Source: CAD feature listing. Evaluate the final solid. Frame: model axes, mm. A direction names the side the tool comes from. Give positions to 0.01 mm unless a question says otherwise; leave off trailing zeros. Write each loop counter-clockwise with the first axis right and the second up, starting at its lowest first coordinate (ties: lowest second). Pieces come first, ordered by that corner, then holes. Notation, with made-up numbers: (-4.75, -29.75) -> (14.25, -29.75) arc R25 cw to (14.25, 9.25) -> close; hole circle Ø3 at (35, -28.5). An arc over 180 degrees is marked (long way). Use one line per item in the form item = value. Start each with the question number.
(1) Material intervals for line 1 along Y through (x, z) = (-18.5, 1.25); line 2 along Y through (x, z) = (-26, 4.25); line 3 along Y through (x, z) = (12, 9.5), sorted ascending. Write a range as from..to.
(2) Cut plane A-A, the plane x = -29. Output: boundary loops of the cut face in (y, z).
(3) Cut plane B-B, the plane z = 3.25. Count the separate pieces of the cut face and the enclosed holes in it, and give its area (3 significant figures).
(4) First-contact query: P1, Ø4, axis at x = -27, z = 4, coming from the +Y side; P2, Ø12, axis at x = 28.5, y = 39.5, coming from the -Z side; P3, Ø1.9, axis at x = -8.5, z = 6, coming from the +Y side; P4, Ø1.6, axis at x = -3.5, z = 7, coming from the +Y side. Flat tips, straight axial feed; report the tip coordinate or a pass-through.
(5) Draft query along Y for faces 1 (the face through (0.399, -9.447, 5.07)), 2 (the face through (0, 50, 5)), 3 (the face through (-7.223, -17.009, 5.07)), 4 (the face through (0, 6, 0)). Return one class per face: pulls with the +Y half, pulls with the -Y half, needs draft (parallel to the pull), parting line crosses it, or undercut.
(6) Set-up query: faces 5 (the face through (-36, 1, 5)), 6 (the face through (-23, 40, 5)), 7 (the face through (7.235, 13.503, 5.07)). Return all of +Z, -Z, +X, -X, +Y, -Y with unobstructed straight access to the full face (end or side cutting, diameter ignored); none if empty.
from build123d import *

# Parameters (mm, degrees)
F1_DEPTH = 10
F2_SIZE  = 1.49999
F4_DEPTH = 10


# Not quite as in the source:
# - a fillet or chamfer is up to 0.001 mm smaller than in the source, because OpenCascade refuses the exact size


with BuildPart() as f1:
    # F0 (on Top) → F1 (new body)
    with BuildSketch(Plane.XY):
        with BuildLine():
            Line((7.0000007749, 40), (10, 40))
            ThreePointArc((10, 40), (0, 50), (-10, 40))
            Line((-10, 40), (-7.0000007749, 40))
            ThreePointArc((-7.0000007749, 40), (0, 47.0000007749), (7.0000007749, 40))
        make_face()
        Polygon((36, -40), (36, 40), (10, 40), (7.0000007749, 40), (-7.0000007749, 40), (-10, 40), (-36, 40), (-36, -40), align=None)
    extrude(amount=F1_DEPTH)

    # F2 (size 1.5 in the source; OpenCascade refuses exactly that, so slightly less here)
    f2_edges = [f1.edges().sort_by_distance(p)[0] for p in [
        (0, 50, 10),
        (-23, 40, 10),
        (-36, 0, 10),
        (0, -40, 10),
        (36, 0, 10),
        (23, 40, 10),
        (0, 47.000001, 10),
        (0, 40, 10),
        (0, 50, 0),
        (-23, 40, 0),
        (-36, 0, 0),
        (0, -40, 0),
        (36, 0, 0),
        (23, 40, 0),
        (0, 47.000001, 0),
        (0, 40, 0),
    ]]
    chamfer(f2_edges, length=F2_SIZE)

    # F3 (on face) → F4 (cut)
    with BuildSketch(Plane.XY.offset(10)):
        Polygon((9.01941, 13.251642), (-7.413878, -15.645048), (9.01941, 1.689704), align=None)
        Polygon((-5.229314, 10.897392), (-0.043674, 10.897392), (2.962569, 11.978135), (5.871741, 13.023694), (8.637504, 13.995209), (11.213521, 14.853819), (13.553455, 15.560666), (15.610967, 16.076888), (16.940888, 16.315581), (18.066333, 16.408794), (18.967754, 16.340134), (19.485045, 16.172547), (19.857078, 15.897769), (20.075875, 15.509104), (20.140122, 15.005391), (19.980223, 14.112285), (19.543063, 13.014817), (18.845257, 11.726576), (17.710823, 9.98186), (16.264623, 8.013275), (14.174175, 5.408678), (11.72632, 2.555867), (8.966951, -0.507624), (5.716937, -3.981084), (2.218444, -7.607146), (-1.472083, -11.339644), (-5.298199, -15.132416), (-9.20346, -18.939297), (-7.467058, -18.939297), (-3.873072, -15.801826), (-0.094887, -12.481081), (3.769463, -9.040146), (7.621943, -5.542107), (11.36452, -2.050048), (14.671952, 1.148161), (17.718542, 4.234917), (20.424586, 7.15893), (22.376178, 9.451811), (23.983998, 11.56327), (25.043446, 13.189903), (25.792536, 14.645471), (26.202411, 15.911404), (26.271608, 16.686717), (26.143923, 17.349851), (25.809161, 17.894215), (25.267338, 18.318258), (24.53297, 18.627591), (23.621676, 18.82837), (21.854292, 18.939297), (19.744262, 18.817766), (17.353663, 18.488244), (14.744575, 17.975197), (11.979075, 17.30309), (8.331078, 16.256236), (4.658259, 15.041801), (1.0886, 13.710223), (-2.249918, 12.31194), align=None)
        Polygon((-5.840144, 17.088177), (-3.619251, 18.933561), (-5.855152, 18.933561), (-7.766318, 17.582905), (-9.890915, 15.963704), (-12.153333, 14.1388), (-14.477963, 12.171034), (-16.789194, 10.123247), (-19.011419, 8.058281), (-20.833308, 6.276802), (-22.476192, 4.573508), (-23.888546, 2.991223), (-24.802964, 1.860788), (-25.518263, 0.852267), (-26.00945, -0.013567), (-26.195816, -0.487065), (-26.271609, -0.886829), (-26.230101, -1.207268), (-26.064565, -1.442791), (-25.726944, -1.601419), (-25.239428, -1.656759), (-24.209316, -1.56342), (-22.607846, -1.213122), (-20.724778, -0.679711), (-18.671706, -0.044733), (-16.560227, 0.610268), (-14.501933, 1.203748), (-13.152533, 1.53891), (-11.922154, 1.776), (-10.849071, 1.887047), (-9.838371, 1.818066), (-9.158572, 1.492121), (-8.872137, 1.070319), (-8.770299, 0.510027), (-8.901347, -0.43259), (-9.311798, -1.573728), (-10.129528, -3.159215), (-11.258734, -4.942681), (-12.651899, -6.877665), (-14.261505, -8.917703), (-16.040031, -11.016334), (-18.545222, -13.775636), (-21.151889, -16.451403), (-23.753323, -18.939297), (-21.841571, -18.939297), (-19.26416, -16.826499), (-16.566892, -14.424306), (-13.846275, -11.824217), (-11.198816, -9.11773), (-9.327369, -7.082132), (-7.590687, -5.076318), (-6.028942, -3.138376), (-4.738285, -1.386829), (-3.678568, 0.235044), (-2.884733, 1.694116), (-2.391719, 2.957258), (-2.24357, 3.715625), (-2.276453, 4.347186), (-2.5028, 4.840154), (-2.934991, 5.182783), (-3.574073, 5.372), (-4.395773, 5.424114), (-6.021186, 5.269587), (-7.929695, 4.890115), (-10.007823, 4.363257), (-12.142089, 3.766577), (-14.219015, 3.177635), (-15.808866, 2.752566), (-17.218733, 2.429106), (-18.505432, 2.241234), (-19.124111, 2.244482), (-19.559671, 2.362015), (-19.803219, 2.624939), (-19.830168, 3.023301), (-19.558342, 3.744641), (-18.971466, 4.657578), (-17.935128, 5.935143), (-16.584765, 7.39239), (-14.985004, 8.983921), (-13.200474, 10.664336), (-10.763992, 12.85997), (-8.266136, 15.032448), align=None)
    extrude(amount=-F4_DEPTH, mode=Mode.SUBTRACT)


solid = f1.part
Geometry says:
q1.line_1 = -39.75..-16.15, -13.73..0.01, 2.24..5.24, 8.53..39.75
q1.line_2 = -40..-1.47, 0..40
q1.line_3 = -39..-1.44, 2.87..15.09, 17.31..39
q2.outline = (-40, 1.5) -> (-38.5, 0) -> (38.5, 0) -> (40, 1.5) -> (40, 8.5) -> (38.5, 10) -> (-38.5, 10) -> (-40, 8.5) -> close
q3.separate_pieces = 1
q3.enclosed_holes = 4
q3.area = 5,350 mm^2
q4.P1 = 40
q4.P2 = 0
q4.P3 = 46.56
q4.P4 = 49.63
q5.face_1 = undercut
q5.face_2 = pulls with the +Y half
q5.face_3 = undercut
q5.face_4 = needs draft
q6.face_5 = +Z, -Z, -X, +Y, -Y
q6.face_6 = +Z, -Z, -X, +Y
q6.face_7 = +Z, -Z
